Model file for the job. Use its own axes, mm. Face numbers are marked on the shaded views. A direction names the side the tool comes from. Round coordinates to 2 decimals unless told otherwise and drop trailing zeros. Write each loop counter-clockwise with the first axis right and the second up, starting at its lowest first coordinate (ties: lowest second). Pieces come first, ordered by that corner, then holes.
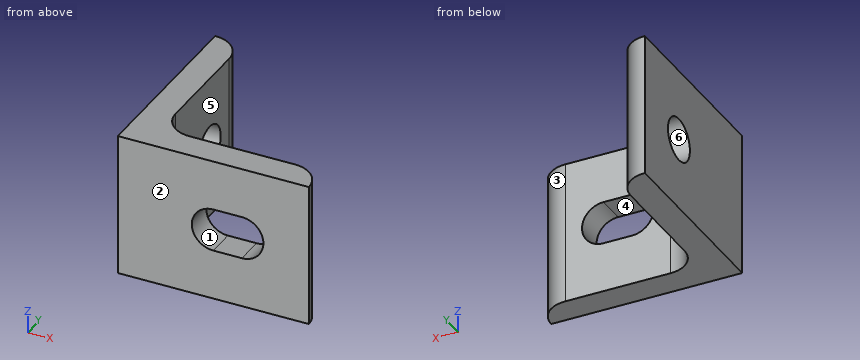
Autodesk Inventor part; units mm, degrees
ref_plane "YZ Plane" through (0, 0, 0) normal (1, 0, 0) x (0, 1, 0)
ref_plane "XZ Plane" through (0, 0, 0) normal (0, 1, 0) x (-1, 0, 0)
ref_plane "XY Plane" through (0, 0, 0) normal (0, 0, 1) x (1, 0, 0)
sketch "スケッチ1" plane through (0, 0, 0) normal (0, 0, 1) x (1, 0, 0)
  line L0 (0, 0) -> (0, 20)
  line L1 (0, 20) -> (3, 20)
  line L2 (3, 20) -> (3, 3)
  line L3 (3, 3) -> (20, 3)
  line L4 (20, 3) -> (20, 0)
  line L5 (20, 0) -> (0, 0)
  dimension "d0" = 3
  dimension "d1" = 3
  dimension "d2" = 20
  dimension "d3" = 20
extrude "押し出し1" add sketch "スケッチ1" along normal blind 15
fillet "フィレット1" radius 3 2 edges at (3, 20, 7.5) (20, 3, 7.5)
sketch "スケッチ2" plane through (0, 0, 0) normal (-1, 0, 0) x (0, 0, 1)
  line L0 (0, 0) -> (0, 20) construction
  line L1 (0, 0) -> (15, 0) construction
  line L2 (15, 20) -> (15, 0) construction
  line L3 (0, 20) -> (15, 20) construction
  circle A0 centre (7.5, 13) radius 2.25
  dimension "d7" = 13
  dimension "d8" = 4.5
  dimension "d9" = 7.5
extrude "押し出し2" cut sketch "スケッチ2" against normal through all
sketch "スケッチ3" plane through (0, 0, 0) normal (0, -1, 0) x (1, 0, 0)
  arc A0 (10, 9.75) -> (10, 5.25) centre (10, 7.5) ccw
  line L0 (10, 7.5) -> (10, 9.75) construction
  line L1 (10, 7.5) -> (12.25, 7.5) construction
  line L2 (10, 7.5) -> (10, 5.25) construction
  arc A1 (13, 5.25) -> (13, 9.75) centre (13, 7.5) ccw
  line L3 (13, 7.5) -> (13, 9.75) construction
  line L4 (13, 7.5) -> (15.25, 7.5) construction
  line L5 (13, 7.5) -> (13, 5.25) construction
  line L6 (10, 9.75) -> (13, 9.75)
  line L7 (0, 15) -> (20, 15)
  line L8 (13, 5.25) -> (10, 5.25)
  line L9 (0, 0) -> (0, 15)
  dimension "d12" = 90
  dimension "d13" = 180
  dimension "d14" = 90
  dimension "d15" = 180
  dimension "d16" = 7.5
  dimension "d17" = 3
  dimension "d18" = 10
  dimension "d19" = 2.25
extrude "押し出し3" cut sketch "スケッチ3" against normal through all
fillet "フィレット2" radius 3 1 edges at (3, 3, 7.5)
properties part number "M4L"
1) Cut at A-A on y = 13. List the corners of the cut face in (x, z), and give its area (3 significant figures).
2) Cut at D-D on y = 2.5. List the corners of the cut face in (x, z).
3) Pull direction X, two halves, no side cores. Call the marked faces 1, 2 and 3: released by +X, released by -X, zero draft, split by the parting line, or undercut.
4) Flat gauge pins, fed straight in: pin 1 Ø4 at (x, z) = (7, 1.5) entering from -Y; pin 2 Ø1.5 at (y, z) = (5.5, 4.5) entering from +X; pin 3 Ø6 at (x, z) = (9.5, 3) entering from +Y; pin 4 Ø5 at (x, y) = (13, 6) entering from +Z. Where does each tip first touch, or does it go through?
5) Wall check: probe 1 along Y at (x, z) = (16, 6); probe 2 along Y at (x, z) = (1.05, 7.5). Give the ranges that are in metal, low to high.
6) Which spindle directions (+Z, -Z, +X, -X, +Y, -Y) get a long thin tool onto all of the face, cutting with end or side? Do the marked faces 4, 5 and 6. Say none if no direction does.
7) Cut at B-B on z = 8.5. Give the number of separate pieces and of enclosed holes in the cut face, and give its area (3 significant figures).
Result sheet:
1. outline: (0, 0) - (3, 0) - (3, 5.25) - (0, 5.25) - close; (0, 9.75) - (3, 9.75) - (3, 15) - (0, 15) - close
1. area: 31.5 mm2
2. outline: (0, 0) - (18.66, 0) - (18.66, 15) - (0, 15) - close; hole (10, 5.25) - (13, 5.25) arc R2.25 ccw to (13, 9.75) - (10, 9.75) arc R2.25 ccw to start
3. face 1: undercut
3. face 2: zero draft
3. face 3: released by +X
4. pin 1: stops at y = 0
4. pin 2: stops at x = 3.27
4. pin 3: stops at y = 3
4. pin 4: passes through
5. probe 1: y = 0 to 3
5. probe 2: y = 0 to 10.75, 15.25 to 19.81
6. face 4: +Y, -Y
6. face 5: +Z, -Z, +X, +Y
6. face 6: +X, -X
7. separate pieces: 3
7. enclosed holes: 0
7. area: 75.9 mm2
